Source: CAD feature listing. Evaluate the final solid. Frame: model axes, mm. A direction names the side the tool comes from. Give positions to 0.01 mm unless a question says otherwise; leave off trailing zeros. Write each loop counter-clockwise with the first axis right and the second up, starting at its lowest first coordinate (ties: lowest second). Pieces come first, ordered by that corner, then holes. Notation, with made-up numbers: (28.25, 35) -> (84.25, 35) arc R20 cw to (84.25, 66) -> close; hole circle Ø4 at (63, 5). An arc over 180 degrees is marked (long way). Answer as a JSON object with one key per item and string values. Group by question number.
Item 1: Section query B-B on z = 10. Return the cut outline in (x, y).
Item 2: Section query D-D on x = -70. Return the cut outline in (y, z), plus the area to 3 significant figures.
Item 3: Section query C-C on y = -2.75. Return the cut outline in (x, z), plus the area to 3 significant figures.
Item 4: Access query for faces 4 (the face through (-9, 0, 2.5)), 5 (the face through (-3, 0, 0)). Directions: +Z, -Z, +X, -X, +Y, -Y. A direction counts if a zero-diameter tool reaches every point of the face in a straight line with its end or side. Return the directions, or none.
Item 5: Pull-direction query (X, two-part tool) for faces 1 (the face through (200, 0, 10)), 2 (the face through (-3, 0, 20)), 3 (the face through (-9, 0, 17.5)); classes: pulls with the +X half, pulls with the -X half, needs draft (parallel to the pull), parting line crosses it, or undercut.
Item 6: Section query A-A on x = 190. Return the cut outline in (y, z), plus the area to 3 significant figures.
Item 7: Ray query, probe 1 along X at (y, z) = (2.25, 10); probe 2 along X at (y, z) = (-3.75, 2.75); probe 3 along X at (y, z) = (0.75, 8.5). Return the intervals inside material, ascending. Write a range as from..to.
from build123d import *

# Parameters (mm, degrees)
SKETCH_1_W          = 400
SKETCH_1_H          = 10
EXTRUDE_1_DEPTH     = 20
SKETCH_2_W          = 250
SKETCH_2_H          = 15
CUT_EXTRUDE_1_DEPTH = 20
SKETCH_4_R          = 5
CUT_EXTRUDE_3_DEPTH = 20


with BuildPart() as part:
    # Эскиз1 → Бобышка-Вытянуть1 (new body)
    with BuildSketch(Plane.XY):
        Rectangle(SKETCH_1_W, SKETCH_1_H)
    extrude(amount=EXTRUDE_1_DEPTH)

    # Эскиз2 → Вырез-Вытянуть1 (cut)
    with BuildSketch(Plane(origin=(0, 5, 0), x_dir=(1, 0, 0), z_dir=(0, 1, 0))):
        with Locations((-7.463718673, -10)):
            Rectangle(SKETCH_2_W, SKETCH_2_H)
    extrude(amount=-CUT_EXTRUDE_1_DEPTH, mode=Mode.SUBTRACT)

    # Эскиз4 → Вырез-Вытянуть3 (cut)
    with BuildSketch(Plane(origin=(0, 5, 0), x_dir=(1, 0, 0), z_dir=(0, 1, 0))):
        with Locations(Location((190, -10, 0), (0, 0, 270))):
            Circle(SKETCH_4_R)
    extrude(amount=-CUT_EXTRUDE_3_DEPTH, mode=Mode.SUBTRACT)


solid = part.part
Worked answers:
{
 "1": {"outline": "(-200, -5) -> (-132.46, -5) -> (-132.46, 5) -> (-200, 5) -> close; (117.54, -5) -> (185, -5) -> (185, 5) -> (117.54, 5) -> close; (195, -5) -> (200, -5) -> (200, 5) -> (195, 5) -> close"},
 "2": {"outline": "(-5, 0) -> (5, 0) -> (5, 2.5) -> (-5, 2.5) -> close; (-5, 17.5) -> (5, 17.5) -> (5, 20) -> (-5, 20) -> close", "area": "50.0 mm^2"},
 "3": {"outline": "(-200, 0) -> (200, 0) -> (200, 20) -> (-200, 20) -> close; hole (-132.46, 2.5) -> (117.54, 2.5) -> (117.54, 17.5) -> (-132.46, 17.5) -> close; hole circle Ø10 at (190, 10)", "area": "4,170 mm^2"},
 "4": {"face 4": "+Y, -Y", "face 5": "-Z, +X, -X, +Y, -Y"},
 "5": {"face 1": "pulls with the +X half", "face 2": "needs draft", "face 3": "undercut"},
 "6": {"outline": "(-5, 0) -> (5, 0) -> (5, 5) -> (-5, 5) -> close; (-5, 15) -> (5, 15) -> (5, 20) -> (-5, 20) -> close", "area": "100 mm^2"},
 "7": {"probe 1": "-200..-132.46, 117.54..185, 195..200", "probe 2": "-200..-132.46, 117.54..200", "probe 3": "-200..-132.46, 117.54..185.23, 194.77..200"}
}
